Here's how the part is built. I have some questions about the finished solid (model axes, mm). Face numbers are marked on the shaded views. A direction names the side the tool comes from. Round coordinates to 2 decimals unless told otherwise and drop trailing zeros. Loops run counter-clockwise (first coordinate to the right, second up) from the corner with the lowest first, then second, coordinate; pieces in that order, holes last. Notation, with made-up numbers: M 63,-9 L 76,-9 A31 cw 76,21 Z; hole C -9.75,6 d5. An arc over 180 degrees is marked long. Put each result on its own line as item: value. Start each with the question number.
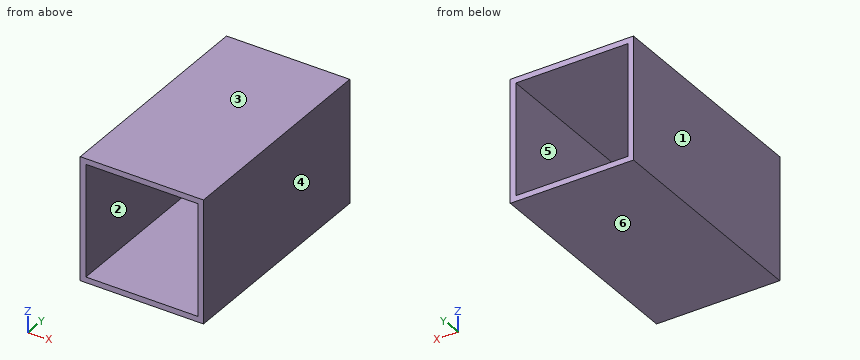
```python
from build123d import *

# Parameters (mm, degrees)
SKETCH_1_W               = 55
SKETCH_1_H               = 55
EXTRUDE_1_DEPTH          = 100
CUT_EXTRUDE_1_DEPTH      = 108.296318669
CUT_EXTRUDE_1_DEPTH_BACK = 108.296318669
SKETCH_2_W               = 50
SKETCH_2_H               = 50


with BuildPart() as part:
    # 草图1 → 凸台-拉伸1 (new body)
    with BuildSketch(Plane(origin=(0, 0, 0), x_dir=(1, 0, 0), z_dir=(0, 1, 0))):
        Rectangle(SKETCH_1_W, SKETCH_1_H)
    extrude(amount=EXTRUDE_1_DEPTH)

    # 草图2 → 切除-拉伸1 (cut, two sides: drawn at the far end of the back side and taken through both)
    with BuildSketch(Plane(origin=(0, 0, 0), x_dir=(1, 0, 0), z_dir=(0, 1, 0)).offset(-CUT_EXTRUDE_1_DEPTH_BACK)):
        Rectangle(SKETCH_2_W, SKETCH_2_H)
    extrude(amount=CUT_EXTRUDE_1_DEPTH + CUT_EXTRUDE_1_DEPTH_BACK, mode=Mode.SUBTRACT)


solid = part.part
```
1) If I drill on probe 1 along X at (y, z) = (83.5, 12), over which ranges is the centre line in solid material (lowest first)? Write a range as from..to.
2) Suppose I cut it at B-B (y = 85.5). Write out the boundary of the cut face in (x, z), plus the area to 3 significant figures.
3) Suppose I cut it at C-C (x = -1). Write out the boundary of the cut face in (y, z), plus the area to 3 significant figures.
4) If we mould it in two halves opening along X, with no side actions, what happens to the marked faces 1, 2, 3 and 4? For each: pulls with the +X half, pulls with the -X half, needs draft (parallel to the pull), parting line crosses it, or undercut.
5) On a 3-axis mill with a long thin cutter (end or side, diameter ignored), from which of +Z, -Z, +X, -X, +Y, -Y can I reach the whole of each face in a straight line? I mean the marked faces 5 and 6. Say none if no direction works.
6) Suppose I cut it at A-A (z = 6). Write out the boundary of the cut face in (x, y).
Results are:
1. probe 1: -27.5..-25, 25..27.5
2. outline: M -27.5,-27.5 L 27.5,-27.5 L 27.5,27.5 L -27.5,27.5 Z; hole M -25,-25 L 25,-25 L 25,25 L -25,25 Z
2. area: 525 mm²
3. outline: M 0,-27.5 L 100,-27.5 L 100,-25 L 0,-25 Z; M 0,25 L 100,25 L 100,27.5 L 0,27.5 Z
3. area: 500 mm²
4. face 1: pulls with the -X half
4. face 2: undercut
4. face 3: needs draft
4. face 4: pulls with the +X half
5. face 5: +Y, -Y
5. face 6: -Z, +X, -X, +Y, -Y
6. outline: M -27.5,0 L -25,0 L -25,100 L -27.5,100 Z; M 25,0 L 27.5,0 L 27.5,100 L 25,100 Z
